Autodesk Inventor part; units mm, degrees
ref_plane "Plano de correa" through (0, 48, 10) normal (0, 0, 1) x (1, 0, 0)
ref_plane "YZ Plane" through (0, 0, 0) normal (1, 0, 0) x (0, 1, 0)
ref_plane "XZ Plane" through (0, 0, 0) normal (0, 1, 0) x (-1, 0, 0)
sketch "Boceto principal" plane through (0, 0, 0) normal (1, 0, 0) x (0, 1, 0)
  line L0 (0, 20) -> (61.8, 20)
  line L1 (61.8, 20) -> (61.8, 16.356)
  line L2 (61.8, 16.356) -> (48, 12.137)
  line L3 (48, 12.137) -> (48, 7.863)
  line L4 (48, 7.863) -> (61.8, 3.644)
  line L5 (61.8, 3.644) -> (61.8, 0)
  line L6 (61.8, 0) -> (0, 0)
  line L7 (59, 15.5) -> (59, 4.5) construction
  line L8 (48, 10) -> (59, 10) construction
  line L9 (61.8, 16.356) -> (61.8, 3.644)
  line L10 (0, -4) -> (0, 24)
  line L11 (0, 0) -> (0, 20)
  dimension "d0" = 11
  dimension "d1" = 34
  dimension "d2" = 2.8
  dimension "d6" = 20
  dimension "d21" = 118
  dimension "d25" = 13.8
  dimension "d27" = 10
ref_plane "Plano de correa" through (0, 48, 10) normal (0, 0, 1) x (1, 0, 0)
revolve "Cuerpo" add sketch "Boceto principal" angle 360 about axis through (0, 0, -10) along (0, 0, 1)
revolve "Para ranuras" cut sketch "Boceto principal" angle 360 about axis through (0, 0, -10) along (0, 0, 1) contours L9 L4 L3 L2
fillet "Empalme externo" [suppressed]
fillet "Empalme interno" [suppressed]
pattern_of_one "Patrón para ranuras"
sketch "Boceto2" plane through (0, 0, 20) normal (0, 0, 1) x (1, 0, 0)
  circle A0 centre (0, 0) radius 22.5
  dimension "d28" = 45
extrude "Extrusión1" cut sketch "Boceto2" against normal blind 30
equation "\"d0\" = da_Bw"
equation "\"d1\" = da_Alfa"
equation "\"d2\" = da_c"
equation "\"d21\" = da_Dw"
equation "\"d25\" = da_Hd"
equation "\"d27\" = da_Se"
equation "\"da_r1\" = 0"
equation "\"da_r2\" = 0"
equation "\"d18\" = da_Sg"
equation "\"da_Bw\" = 11"
equation "\"da_Alfa\" = 34deg"
equation "\"da_c\" = 2.8"
equation "\"da_Dw\" = 118"
equation "\"da_Hd\" = 13.8"
equation "\"da_Se\" = 10"
equation "\"da_Sg\" = 15"
properties part number "Polea ranurada1" material "Steel"
Here's how the part is built. I have some questions about the finished solid (model axes, mm). A direction names the side the tool comes from. Give positions to 0.01 mm unless a question says otherwise; leave off trailing zeros. Loops run counter-clockwise (first coordinate to the right, second up) from the corner with the lowest first, then second, coordinate; pieces in that order, holes last. Notation, with made-up numbers: (39.25, -29) -> (81.25, -29) arc R10 ccw to (81.25, -12) -> close; hole circle Ø3 at (22, -5). An arc over 180 degrees is marked (long way). Answer as a JSON object with one key per item and string values. Group by question number.
Item 1: Imagine slicing it at A-A on x = 0. Write out the boundary of the cut face in (y, z), then the cut area to 3 significant figures.
Item 2: I need wall thicknesses on L1, parallel to Y at x = 18, z = 9.75; L2, parallel to Y at x = -12, z = 18.25; L3, parallel to Z at x = 10.5, y = 49. Which ranges of each line are inside material? Lowest first, please.
Item 3: On a 3-axis mill with a long thin cutter (end or side, diameter ignored), from which of +Z, -Z, +X, -X, +Y, -Y can I reach the whole of each face in a straight line? I mean faces 4 (the conical face through (-47.7, -10.6, 7.6)), 5 (the cylindrical face through (-37.604, -49.042, 1.796)). Say none if no direction works.
Item 4: Thinking about a two-plate mould opening in X: for faces 1 (the flat face through (-1, 27, 0)), 2 (the cylindrical face through (2.11, -47.954, 9.97)), 3 (the cylindrical face through (10.382, -19.961, 10.14)), which applies, pulls with the +X half, pulls with the -X half, needs draft (parallel to the pull), parting line crosses it, or undercut?
Item 5: Imagine slicing it at D-D on z = 6. Write out the boundary of the cut face in (x, y), then the cut area to 3 significant figures.
Item 6: Imagine slicing it at C-C on z = 18.25. Write out the boundary of the cut face in (x, y), then the cut area to 3 significant figures.
Item 7: Will these pins go through, and if not, where does the flat tip stop? pin 1 (10 mm diameter, centred on y = 5, z = 11.5, fed in from -X); pin 2 (8 mm diameter, centred on y = 23.5, z = 15, fed in from +X); pin 3 (2 mm diameter, centred on x = -35, z = 4.5, fed in from +Y).
Answer list:
{
 "1": {"outline": "(-61.8, 0) -> (-22.5, 0) -> (-22.5, 20) -> (-61.8, 20) -> (-61.8, 16.36) -> (-48, 12.14) -> (-48, 7.86) -> (-61.8, 3.64) -> close; (22.5, 0) -> (61.8, 0) -> (61.8, 3.64) -> (48, 7.86) -> (48, 12.14) -> (61.8, 16.36) -> (61.8, 20) -> (22.5, 20) -> close", "area": "1,340 mm2"},
 "2": {"L1": "y = -44.5 to -13.5, 13.5 to 44.5", "L2": "y = -60.62 to -19.03, 19.03 to 60.62", "L3": "z = 0 to 7.22, 12.78 to 20"},
 "3": {"face 4": "none", "face 5": "+Z, -Z"},
 "4": {"face 1": "needs draft", "face 2": "parting line crosses it", "face 3": "undercut"},
 "5": {"outline": "circle Ø108.19 at (0, 0); hole circle Ø45 at (0, 0)", "area": "7,600 mm2"},
 "6": {"outline": "circle Ø123.6 at (0, 0); hole circle Ø45 at (0, 0)", "area": "10,400 mm2"},
 "7": {"pin 1": "stops at x = -61.68", "pin 2": "stops at x = 58.56", "pin 3": "stops at y = 51.29"}
}
